```python
from build123d import *

# Parameters (mm, degrees)
F0_R     = 50.8
F0_R_2   = 10.16
F1_DEPTH = 6.35
F2_SIZE  = 3.175
F3_SIZE  = 3.17499


# Not quite as in the source:
# - a fillet or chamfer is up to 0.001 mm smaller than in the source, because OpenCascade refuses the exact size


with BuildPart() as f1:
    # F0 (on Front) → F1 (new body)
    with BuildSketch(Plane.XZ):
        Circle(F0_R)
        Circle(F0_R_2, mode=Mode.SUBTRACT)
    extrude(amount=F1_DEPTH)

    # F2
    f2_edges = [f1.edges().sort_by_distance(p)[0] for p in [
        (-50.8, -6.35, 0),
    ]]
    chamfer(f2_edges, length=F2_SIZE)

    # F3 (size 3.175 in the source; OpenCascade refuses exactly that, so slightly less here)
    f3_edges = [f1.edges().sort_by_distance(p)[0] for p in [
        (-50.8, 0, 0),
    ]]
    chamfer(f3_edges, length=F3_SIZE)


solid = f1.part
```
Read the model definition and answer for the solid it produces. Units are mm, in the model's axes. Give positions to 0.01 mm unless a question says otherwise; leave off trailing zeros. Order: outer loops, then holes, each group sorted by start corner. A loop starts at its lowest first (then second) coordinate and runs counter-clockwise, first axis right, second up. Notation, with made-up numbers: (86.5, 75.5) -> (138.5, 75.5) arc R9 cw to (138.5, 80.5) -> close; hole circle Ø4 at (25.5, -4.75). An arc over 180 degrees is marked (long way). One line per item, written item: value. Start each with the question number.
(1) Straight lines are drawn through the part: L1, parallel to X at y = -5.5, z = -3.5; L2, parallel to Z at x = 0, y = -4.5 (3 decimals); L3, parallel to Z at x = 0, y = -3.25 (3 decimals). For each, find the intervals that lie inside material, in ascending order.
(2) For a pull along Z with two mould halves and no side action, classify faces 1 (the cylindrical face through (-1.323, -3.131, 10.074)), 2 (the flat face through (-1, -6.35, 11)), 3 (the conical face through (45.57, -0.15, 14.35)) as released by +Z, released by -Z, zero draft, split by the parting line, or undercut.
(3) Flat-ended cylindrical pins translate along their axes: P1, Ø1, axis at x = -29.5, y = -4.5, coming from the +Z side; P2, Ø2, axis at y = -1, z = 18.5, coming from the +X side; P3, Ø2, axis at x = 1, y = -1.5, coming from the +Z side. Find the tip coordinate at first contact, or state that the pin passes through.
(4) The part is cut by section C-C (y = -4.5). Determine the outline of the cut face in (x, z) (3 decimals), and give its area (3 significant figures).
Taken from the geometry:
1. L1: -48.35 to -9.54, 9.54 to 48.35
1. L2: -49.475 to -10.16, 10.16 to 49.475
1. L3: -50.725 to -10.16, 10.16 to 50.725
2. face 1: undercut
2. face 2: zero draft
2. face 3: split by the parting line
3. P1: z = 40.44
3. P2: x = 46.12
3. P3: z = 50.12
4. outline: circle Ø98.95 at (0, 0); hole circle Ø20.32 at (0, 0)
4. area: 7,370 mm^2
